Here's how the part is built. I have some questions about the finished solid (model axes, mm). Round coordinates to 2 decimals unless told otherwise and drop trailing zeros. Write each loop counter-clockwise with the first axis right and the second up, starting at its lowest first coordinate (ties: lowest second). Pieces come first, ordered by that corner, then holes. Notation, with made-up numbers: (87.5, 82) - (124.5, 82) arc R37 ccw to (124.5, 118) - close; hole circle Ø4 at (-4, -29). An arc over 180 degrees is marked (long way). Use one line per item in the form item = value. Start each with the question number.
1. We'd pull the mould along Y, two halves only. Please class faces 1 (the flat face through (0, -3, 8.35)), 2 (the cylindrical face through (-0.59, 4.46, 4.12)), 3 (the cylindrical face through (1.18, -2.26, 4.12)): +Y half, -Y half, draft (parallel to the pull), parting line (faces both ways), or undercut.
2. I want a section at C-C, the plane z = 1.5. List the corners of the cut face in (x, y) for me, plus the area to 3 significant figures.
3. If I drill on line 1 along Y through (x, z) = (0, 2.5); line 2 along Y through (x, z) = (-1.25, 6); line 3 along X through (y, z) = (0.75, 6), over which ranges is the centre line in solid material (lowest first)?
4. I want a section at A-A, the plane x = 0. List the corners of the cut face in (y, z) for me.
5. Will this pin go through, and if not, where does the flat tip stop? pin 1 (2 mm diameter, centred on y = 2.5, z = 4.5, fed in from +X).
```python
from build123d import *

# Parameters (mm, degrees)
SKETCH1_R           = 4.5
BOSS_EXTRUDE1_DEPTH = 8.35
SKETCH2_R           = 2.55
CUT_EXTRUDE1_DEPTH  = 11.498690395
CHAMFER1_SIZE       = 0.5


with BuildPart() as part:
    # Sketch1 → Boss-Extrude1 (new body)
    with BuildSketch(Plane.XY):
        Circle(SKETCH1_R)
    extrude(amount=BOSS_EXTRUDE1_DEPTH)

    # Sketch2 → Cut-Extrude1 (cut, through all)
    with BuildSketch(Plane.XY):
        Circle(SKETCH2_R)
    extrude(amount=CUT_EXTRUDE1_DEPTH, mode=Mode.SUBTRACT)

    # Chamfer1
    chamfer1_edges = [part.edges().sort_by_distance(p)[0] for p in [
        (-4.5, 0, 0),
        (-4.5, 0, 8.35),
    ]]
    chamfer(chamfer1_edges, length=CHAMFER1_SIZE)


solid = part.part
```
Model answer:
q1.face_1 = draft
q1.face_2 = parting line
q1.face_3 = undercut
q2.outline = circle Ø9 at (0, 0); hole circle Ø5.1 at (0, 0)
q2.area = 43.2 mm2
q3.line_1 = -4.5 to -2.55, 2.55 to 4.5
q3.line_2 = -4.32 to -2.22, 2.22 to 4.32
q3.line_3 = -4.44 to -2.44, 2.44 to 4.44
q4.outline = (-4.5, 0.5) - (-4, 0) - (-2.55, 0) - (-2.55, 8.35) - (-4, 8.35) - (-4.5, 7.85) - close; (2.55, 0) - (4, 0) - (4.5, 0.5) - (4.5, 7.85) - (4, 8.35) - (2.55, 8.35) - close
q5.pin_1 = 4.24
